Build history of the part. All positions in model axes, mm. A direction names the side the tool comes from. Give positions to 0.01 mm unless a question says otherwise; leave off trailing zeros. Write each loop counter-clockwise with the first axis right and the second up, starting at its lowest first coordinate (ties: lowest second). Pieces come first, ordered by that corner, then holes. Notation, with made-up numbers: M 18,19.5 L 68,19.5 A34 cw 68,54.5 Z; hole C -35,32.25 d3. An arc over 180 degrees is marked long. Return JSON: item names as keys, results as strings. Group by question number.
Q1. Wall check: probe 1 along X at (y, z) = (-0.75, -17); probe 2 along Y at (x, z) = (204.5, 2); probe 3 along Z at (x, y) = (185.5, 1.75). Give the ranges that are in metal, low to high.
Q2. Band-saw the part on A-A, the plane x = 125. Give the cut face in (y, z).
Q3. Flat gauge pins, fed straight in: pin 1 Ø9.5 at (x, z) = (144.5, 1) entering from +Y; pin 2 Ø2 at (x, y) = (160.5, 5.5) entering from +Z; pin 3 Ø2 at (x, y) = (88, -1.5) entering from +Z. Where does each tip first touch, or does it go through?
Q4. Tool access for faces 5 (the flat face through (113.75, 0, -14)), 6 (the flat face through (0, 6, 1)), 7 (the flat face through (3, 13.632, 0)): list every direction of +Z, -Z, +X, -X, +Y, -Y with a clear straight run to the whole face (end or side of a thin tool).
Q5. Pull direction Y, two halves, no side cores. Call faces 1 (the flat face through (250, 6, 6)), 2 (the flat face through (123, 6, 0)), 3 (the cylindrical face through (127.54, 0.46, -17.75)), 4 (the flat face through (126, -2.5, -4)): +Y half, -Y half, draft (parallel to the pull), parting line (faces both ways), or undercut.
Q6. Band-saw the part on C-C, the plane z = -7. Give the cut face in (x, y), then the cut area to 3 significant figures.
Q7. Band-saw the part on B-B, the plane x = 16.5. Give the cut face in (y, z), then the cut area to 3 significant figures.
from build123d import *

# Parameters (mm, degrees)
BOSS_EXTRUDE1_DEPTH = 250
SKETCH16_W          = 22.5
SKETCH16_H          = 25.4
SKETCH16_R          = 1.175
SKETCH16_R_2        = 2.75
BOSS_EXTRUDE4_DEPTH = 6
SKETCH17_W          = 22.5
SKETCH17_H          = 6
CUT_EXTRUDE10_DEPTH = 2.5
SKETCH20_W          = 26
SKETCH20_H          = 16
BOSS_EXTRUDE7_DEPTH = 2.5
CUT_EXTRUDE12_DEPTH = 2.5
SKETCH22_W          = 10
SKETCH22_H          = 10
CUT_EXTRUDE13_DEPTH = 10
SKETCH23_W          = 5.437321705
SKETCH23_H          = 8.7625
CUT_EXTRUDE14_DEPTH = 1.25
SKETCH24_W          = 26
SKETCH24_H          = 16
BOSS_EXTRUDE8_DEPTH = 2.5
FILLET1_R           = 2.5


with BuildPart() as part:
    # Sketch1 → Boss-Extrude1 (new body)
    with BuildSketch(Plane.YZ):
        Polygon((0, 4.7625), (-2.5, 4.7625), (-2.5, -4), (14.8825, -4), (14.8825, 4.7625), (12.3825, 4.7625), (12.3825, 0), (0, 0), align=None)
    extrude(amount=BOSS_EXTRUDE1_DEPTH)

    # Sketch16 → Boss-Extrude4 (add)
    with BuildSketch(Plane.XZ.offset(2.5)):
        with Locations((125, -16.7)):
            Rectangle(SKETCH16_W, SKETCH16_H)
        with Locations((117.0625, -16.7)):
            Circle(SKETCH16_R, mode=Mode.SUBTRACT)
        with Locations((132.9375, -16.7)):
            Circle(SKETCH16_R, mode=Mode.SUBTRACT)
        with Locations((125, -16.7)):
            Circle(SKETCH16_R_2, mode=Mode.SUBTRACT)
    extrude(amount=-BOSS_EXTRUDE4_DEPTH)

    # Sketch17 → Cut-Extrude10 (cut)
    with BuildSketch(Plane(origin=(0, 0, -29.4), x_dir=(1, 0, 0), z_dir=(0, 0, -1))):
        with Locations((125, -0.5)):
            Rectangle(SKETCH17_W, SKETCH17_H)
    extrude(amount=-CUT_EXTRUDE10_DEPTH, mode=Mode.SUBTRACT)

    # Sketch20 → Boss-Extrude7 (add)
    with BuildSketch(Plane(origin=(0, 0, 0), x_dir=(0, -1, 0), z_dir=(-1, 0, 0))):
        with Locations((-6.19125, 4)):
            Rectangle(SKETCH20_W, SKETCH20_H)
    extrude(amount=BOSS_EXTRUDE7_DEPTH)

    # Sketch21 → Cut-Extrude12 (cut)
    with BuildSketch(Plane(origin=(-2.5, 0, 0), x_dir=(0, -1, 0), z_dir=(-1, 0, 0))):
        with BuildLine():
            Line((-14.99125, 9), (-14.99125, 0.5))
            ThreePointArc((-14.99125, 0.5), (-16.19125, -0.7), (-17.39125, 0.5))
            Line((-17.39125, 0.5), (-17.39125, 9))
            ThreePointArc((-17.39125, 9), (-16.19125, 10.2), (-14.99125, 9))
        make_face()
        with BuildLine():
            Line((2.60875, 9), (2.60875, 0.5))
            ThreePointArc((2.60875, 0.5), (3.80875, -0.7), (5.00875, 0.5))
            Line((5.00875, 0.5), (5.00875, 9))
            ThreePointArc((5.00875, 9), (3.80875, 10.2), (2.60875, 9))
        make_face()
    extrude(amount=-CUT_EXTRUDE12_DEPTH, mode=Mode.SUBTRACT)

    # Sketch22 → Cut-Extrude13 (cut)
    with BuildSketch(Plane(origin=(-2.5, 0, 0), x_dir=(0, -1, 0), z_dir=(-1, 0, 0))):
        with Locations((-6.19125, 7)):
            Rectangle(SKETCH22_W, SKETCH22_H)
    extrude(amount=-CUT_EXTRUDE13_DEPTH, mode=Mode.SUBTRACT)

    # Sketch23 → Cut-Extrude14 (cut)
    with BuildSketch(Plane(origin=(0, 14.8825, 0), x_dir=(-1, 0, 0), z_dir=(0, 1, 0))):
        with Locations((-2.718660853, 0.38125)):
            Rectangle(SKETCH23_W, SKETCH23_H)
    cut_extrude14 = extrude(amount=-CUT_EXTRUDE14_DEPTH, mode=Mode.SUBTRACT)

    # Mirror8: Cut-Extrude14 across plane
    add(cut_extrude14.mirror(Plane.ZX.offset(6.19125)), mode=Mode.SUBTRACT)

    # Sketch24 → Boss-Extrude8 (add)
    with BuildSketch(Plane.YZ.offset(250)):
        with Locations((6.19125, 4)):
            Rectangle(SKETCH24_W, SKETCH24_H)
    extrude(amount=BOSS_EXTRUDE8_DEPTH)

    # Fillet1
    fillet1_edges = [part.edges().sort_by_distance(p)[0] for p in [
        (136.25, 0.5, -26.9),
        (113.75, 0.5, -26.9),
    ]]
    fillet(fillet1_edges, radius=FILLET1_R)


solid = part.part
From the geometry:
{
 "1": {"probe 1": "x = 113.75 to 115.93, 118.2 to 122.27, 127.73 to 131.8, 134.07 to 136.25", "probe 2": "y = -2.5 to 0, 12.38 to 14.88", "probe 3": "z = -4 to 0"},
 "2": {"outline": "M -2.5,-26.9 L 3.5,-26.9 L 3.5,-19.45 L -2.5,-19.45 Z; M -2.5,-13.95 L 3.5,-13.95 L 3.5,-4 L 14.88,-4 L 14.88,4.76 L 12.38,4.76 L 12.38,0 L 0,0 L 0,4.76 L -2.5,4.76 Z"},
 "3": {"pin 1": "stops at y = 14.88", "pin 2": "stops at z = 0", "pin 3": "stops at z = 4.76"},
 "4": {"face 5": "-Z, -X, +Y, -Y", "face 6": "+Z", "face 7": "+Z, -Z, +Y"},
 "5": {"face 1": "undercut", "face 2": "undercut", "face 3": "draft", "face 4": "-Y half"},
 "6": {"outline": "M 113.75,-2.5 L 136.25,-2.5 L 136.25,3.5 L 113.75,3.5 Z", "area": "135 mm^2"},
 "7": {"outline": "M -2.5,-4 L 14.88,-4 L 14.88,4.76 L 12.38,4.76 L 12.38,0 L 0,0 L 0,4.76 L -2.5,4.76 Z", "area": "93.3 mm^2"}
}
